Verification items for this drawing (mm, ordinates from the low corner). A direction names the side the tool comes from. Round coordinates to 2 decimals unless told otherwise and drop trailing zeros. Write each loop counter-clockwise with the first axis right and the second up, starting at its lowest first coordinate (ties: lowest second). Pieces come first, ordered by that corner, then holes. Notation, with made-up numbers: M -11,79.25 L -2,79.25 A33 cw -2,108.25 Z; hole C 13.5,72 d7. An arc over 180 degrees is marked long. One line per question, with ' | ' between items. Start each with the question number.
Q1. Thickness scan on line 1 along X through (y, z) = (5.5, 9); line 2 along Y through (x, z) = (48.5, 26.5); line 3 along Y through (x, z) = (68, 25). Record the ranges inside material, lowest first. Write a range as from..to.
Q2. Cross-section at C-C (y = 56). Record the boundary of the cut face in (x, z), then the cut area to 3 significant figures.
Q3. Release check for a two-part mould opening along X. For the marked faces 4, 5 and 6 record: released by +X, released by -X, zero draft, split by the parting line, or undercut.
Q4. Tool access check on the marked faces 1, 2 and 3. Record the directions out of +Z, -Z, +X, -X, +Y, -Y that give a thin tool (end or side, any length) a straight path to the whole face; none if there is none.
Q5. Cross-section at D-D (x = 51). Record the boundary of the cut face in (y, z), then the cut area to 3 significant figures.
Q6. Cross-section at A-A (y = 30). Record the boundary of the cut face in (x, z).
Q7. Gauge pin test, flat ends, axial feed: pin 1 (6 mm diameter, centred on x = 8, y = 34.5, fed in from -Z); pin 2 (8 mm diameter, centred on x = 50, z = 34, fed in from -Y). Record the tip position at first contact, or that the pin passes through.
Q8. Cross-section at B-B (z = 25). Record the boundary of the cut face in (x, y).
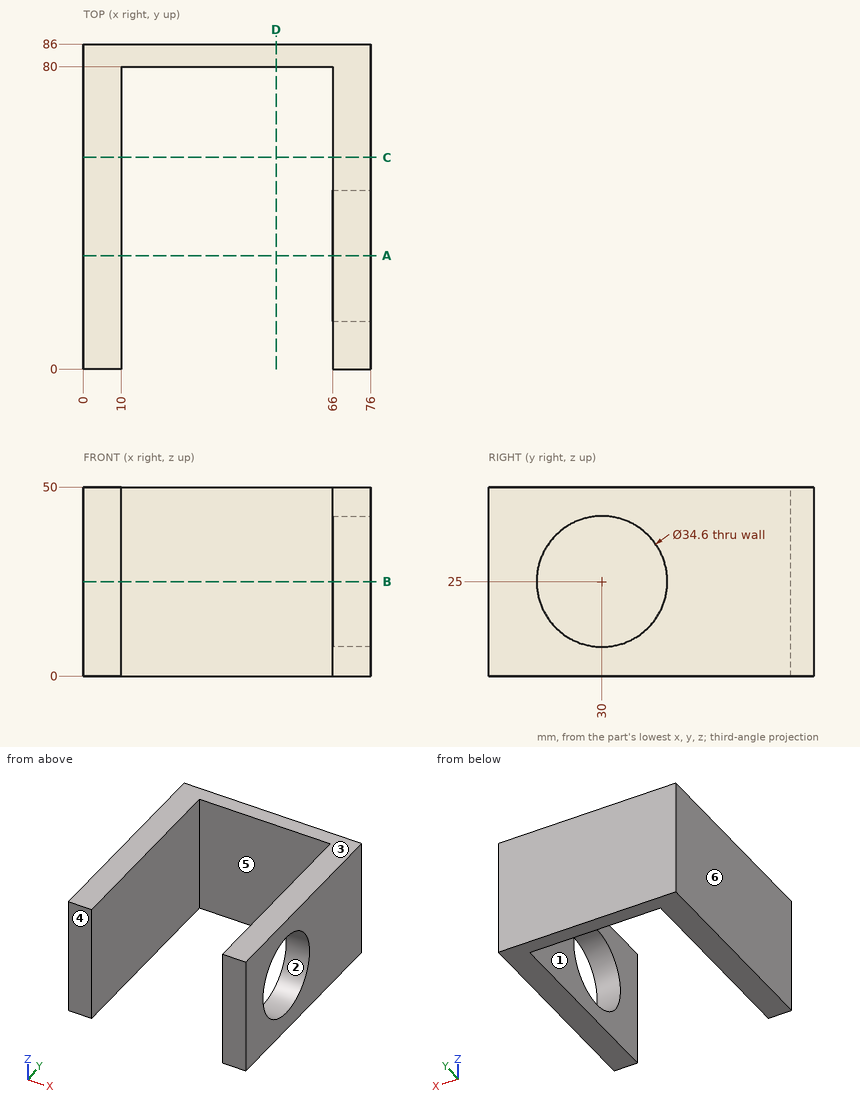
Determined:
1) line 1: x = 0..10, 66..76 | line 2: y = 80..86 | line 3: y = 0..12.7, 47.3..86
2) outline: M 0,0 L 10,0 L 10,50 L 0,50 Z; M 66,0 L 76,0 L 76,50 L 66,50 Z | area: 1,000 mm²
3) face 4: zero draft | face 5: undercut | face 6: released by -X
4) face 1: +Z, -Z, -Y | face 2: +X | face 3: +Z, +X, -X, +Y, -Y
5) outline: M 80,0 L 86,0 L 86,50 L 80,50 Z | area: 300 mm²
6) outline: M 0,0 L 10,0 L 10,50 L 0,50 Z; M 66,0 L 76,0 L 76,7.7 L 66,7.7 Z; M 66,42.3 L 76,42.3 L 76,50 L 66,50 Z
7) pin 1: stops at z = 0 | pin 2: stops at y = 80
8) outline: M 0,0 L 10,0 L 10,80 L 66,80 L 66,47.3 L 76,47.3 L 76,86 L 0,86 Z; M 66,0 L 76,0 L 76,12.7 L 66,12.7 Z
